Check sheet for the drawn part. Datum: minimum x, y, z corner. Units: mm. A direction names the side the tool comes from. Give positions to 0.01 mm unless a question says otherwise; leave off trailing zeros. Order: outer loops, then holes, each group sorted by start corner. A loop starts at its lowest first (then second) coordinate and runs counter-clockwise, first axis right, second up. Notation, with made-up numbers: (82.25, -14) -> (92.25, -14) arc R25 cw to (92.25, 15) -> close; hole circle Ø10 at (19, -38.75). An arc over 180 degrees is marked (long way). Return JSON: item names as keys, results as strings. Group by question number.
(1) Cross-section at D-D on z = 17.5. Enter the section's corners in (x, y), then the cut area to 3 significant figures.
(2) Release check for a two-part mould opening along Z. For the marked faces 3, 4, 5 and 6 record: pulls with the +Z half, pulls with the -Z half, needs draft (parallel to the pull), parting line crosses it, or undercut.
(3) Cross-section at A-A on z = 9.5. Enter the section's corners in (x, y).
(4) Cross-section at C-C on x = 9.5. Enter the section's corners in (y, z), then the cut area to 3 significant figures.
(5) Thickness scan on line 1 along X through (y, z) = (3.1, 9.5); line 2 along X through (y, z) = (11, 26). Record the ranges inside material, lowest first.
(6) Cross-section at B-B on y = 8.75. Enter the section's corners in (x, z).
(7) Tool access check on the marked faces 1 and 2. Record the directions out of +Z, -Z, +X, -X, +Y, -Y that give a thin tool (end or side, any length) a straight path to the whole face; none if there is none.
(8) Depth check by flat-ended pin: pin 1 Ø5.5 at (x, z) = (3.5, 41.5) entering from -Y; pin 2 Ø2 at (x, z) = (20.5, 40) entering from +Y. Enter the tip coordinate at first touch or a pass-through.
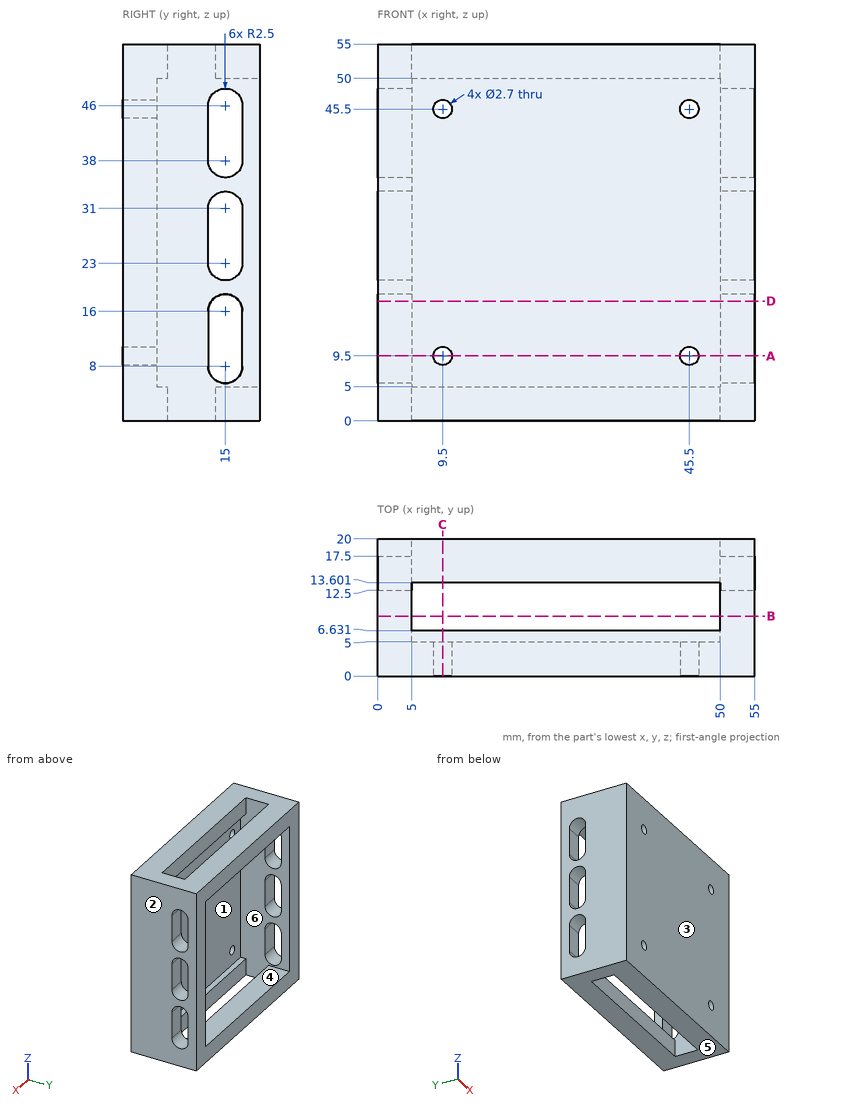
Verdict:
{
 "1": {"outline": "(0, 0) -> (55, 0) -> (55, 13) -> (50, 13) -> (50, 5) -> (5, 5) -> (5, 13) -> (0, 13) -> close; (0, 17) -> (5, 17) -> (5, 20) -> (0, 20) -> close; (50, 17) -> (55, 17) -> (55, 20) -> (50, 20) -> close", "area": "385 mm²"},
 "2": {"face 3": "needs draft", "face 4": "undercut", "face 5": "pulls with the -Z half", "face 6": "undercut"},
 "3": {"outline": "(0, 0) -> (8.15, 0) -> (8.15, 5) -> (5, 5) -> (5, 12.5) -> (0, 12.5) -> close; (0, 17.5) -> (5, 17.5) -> (5, 20) -> (0, 20) -> close; (10.85, 0) -> (44.15, 0) -> (44.15, 5) -> (10.85, 5) -> close; (46.85, 0) -> (55, 0) -> (55, 12.5) -> (50, 12.5) -> (50, 5) -> (46.85, 5) -> close; (50, 17.5) -> (55, 17.5) -> (55, 20) -> (50, 20) -> close"},
 "4": {"outline": "(0, 0) -> (6.63, 0) -> (6.63, 5) -> (5, 5) -> (5, 8.15) -> (0, 8.15) -> close; (0, 10.85) -> (5, 10.85) -> (5, 44.15) -> (0, 44.15) -> close; (0, 46.85) -> (5, 46.85) -> (5, 50) -> (6.63, 50) -> (6.63, 55) -> (0, 55) -> close; (13.6, 0) -> (20, 0) -> (20, 5) -> (13.6, 5) -> close; (13.6, 50) -> (20, 50) -> (20, 55) -> (13.6, 55) -> close", "area": "328 mm²"},
 "5": {"line 1": "0 to 8.15, 10.85 to 44.15, 46.85 to 55", "line 2": "0 to 5, 50 to 55"},
 "6": {"outline": "(0, 0) -> (5, 0) -> (5, 55) -> (0, 55) -> close; (50, 0) -> (55, 0) -> (55, 55) -> (50, 55) -> close"},
 "7": {"face 1": "+Y", "face 2": "+Z, -Z, +X, +Y, -Y"},
 "8": {"pin 1": "y = 0", "pin 2": "y = 5"}
}
